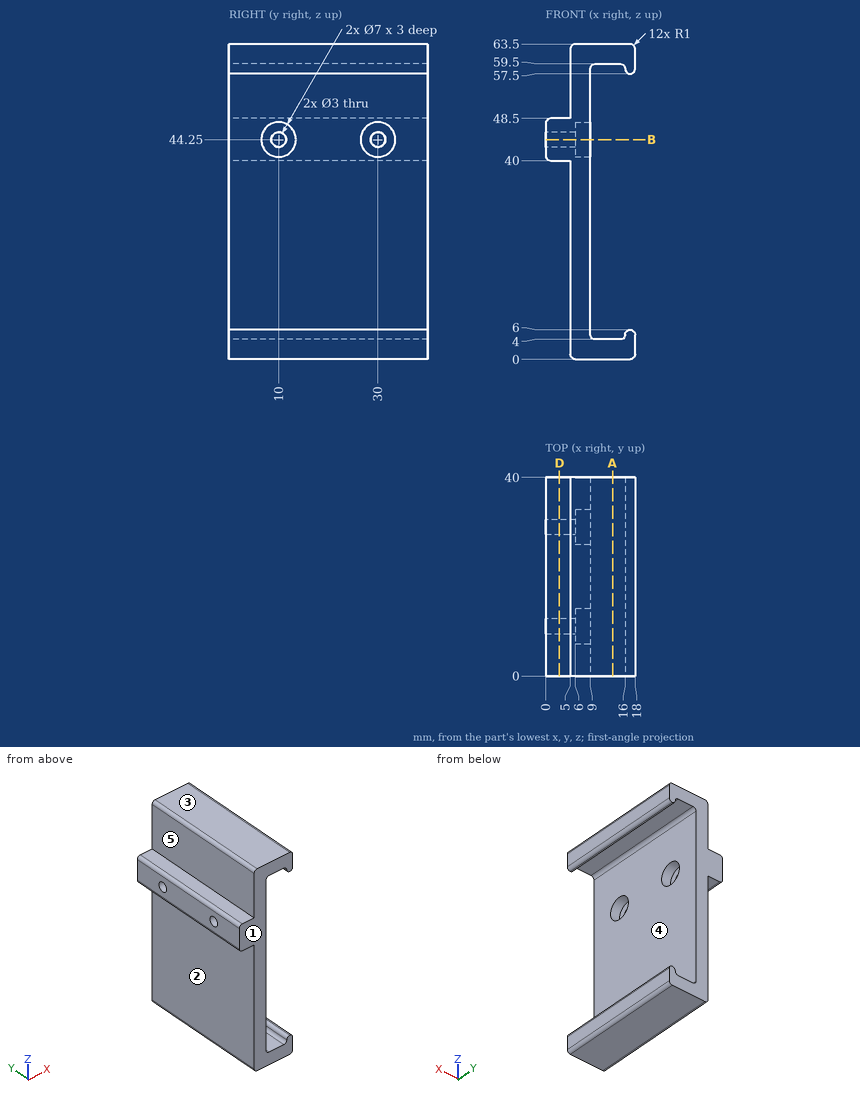
Input: dimensioned drawing with shaded views. Units: mm. Origin: part minimum x, y, z. A direction names the side the tool comes from. Coordinates: 2 decimals unless noted, no trailing zeros. Loops run counter-clockwise (first coordinate to the right, second up) from the corner with the lowest first, then second, coordinate; pieces in that order, holes last. Notation, with made-up numbers: M 57,49.5 L 80,49.5 A23 ccw 80,70.5 Z; hole C 89.5,62.25 d5. An arc over 180 degrees is marked long. Use a Markdown table: item, result. Add a question column.
1) Section D-D, the plane x = 2.75. Return the cut outline in (y, z), plus the area to 3 significant figures.
2) Section A-A, the plane x = 13.5. Return the cut outline in (y, z).
3) Pin query (flat end, axial travel): P1, Ø7.5, axis at y = 11, z = 44, coming from the +X side; P2, Ø5.5, axis at y = 30, z = 44.25, coming from the +X side; P3, Ø4.5, axis at x = 3, y = 29, coming from the -Z side. Return the tip coordinate at first contact, or that it passes through.
4) Draft query along Z for the marked faces 3, 4 and 5. Return one class per face: +Z half, -Z half, draft (parallel to the pull), parting line (faces both ways), or undercut.
5) Section B-B, the plane z = 44.25. Return the cut outline in (x, y).
6) Line query: L1, parallel to Y at x = 1.6, z = 44.25; L2, parallel to Z at x = 10.25, y = 11; L3, parallel to Z at x = 2.8, y = 30. Output: solid intervals per line, ascending. Write a range as from..to.
7) Set-up query: the marked faces 1 and 2. Return all of +Z, -Z, +X, -X, +Y, -Y with unobstructed straight access to the full face (end or side cutting, diameter ignored); none if empty.
Answer below:
| question | item | result |
|---|---|---|
| 1 | outline | M 0,40 L 40,40 L 40,48.5 L 0,48.5 Z; hole C 10,44.25 d3; hole C 30,44.25 d3 |
| 1 | area | 326 mm2 |
| 2 | outline | M 0,0 L 40,0 L 40,4 L 0,4 Z; M 0,59.5 L 40,59.5 L 40,63.5 L 0,63.5 Z |
| 3 | P1 | x = 9 |
| 3 | P2 | x = 6 |
| 3 | P3 | z = 0.34 |
| 4 | face 3 | +Z half |
| 4 | face 4 | undercut |
| 4 | face 5 | draft |
| 5 | outline | M 0,0 L 9,0 L 9,6.5 L 6,6.5 L 6,8.5 L 0,8.5 Z; M 0,11.5 L 6,11.5 L 6,13.5 L 9,13.5 L 9,26.5 L 6,26.5 L 6,28.5 L 0,28.5 Z; M 0,31.5 L 6,31.5 L 6,33.5 L 9,33.5 L 9,40 L 0,40 Z |
| 6 | L1 | 0..8.5, 11.5..28.5, 31.5..40 |
| 6 | L2 | 0..4, 59.5..63.5 |
| 6 | L3 | 40..42.75, 45.75..48.5 |
| 7 | face 1 | +Z, -Z, +X, -X, -Y |
| 7 | face 2 | -Z, -X, +Y, -Y |
